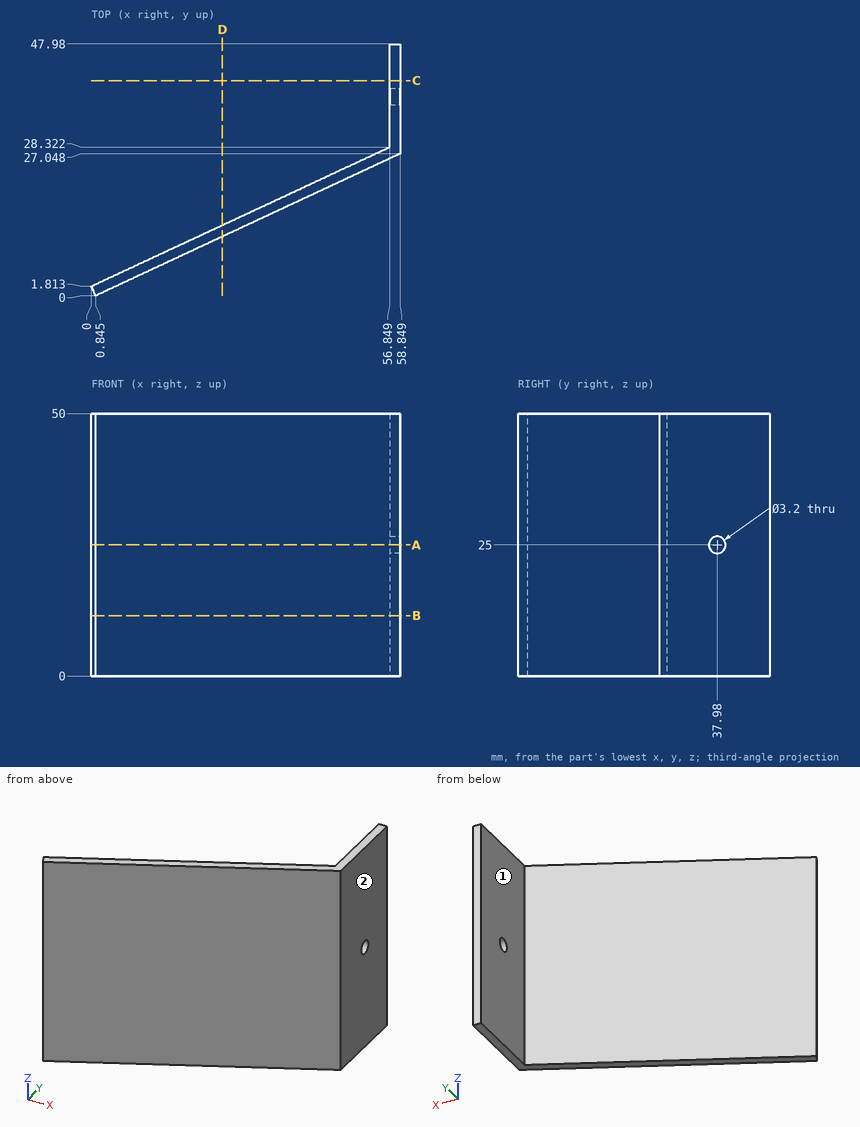
Input: dimensioned drawing with shaded views. Units: mm. Origin: part minimum x, y, z. A direction names the side the tool comes from. Coordinates: 2 decimals unless noted, no trailing zeros. Loops run counter-clockwise (first coordinate to the right, second up) from the corner with the lowest first, then second, coordinate; pieces in that order, holes last. Notation, with made-up numbers: M -3.5,50.25 L 14.5,50.25 A20 cw 14.5,66.25 Z; hole C 80,-16.5 d6. An arc over 180 degrees is marked long. One line per item, written item: value. Start each with the question number.
1) Cut plane D-D (x = 25). Return loops of the section in (y, z), then the cut area to 3 significant figures.
2) Cut plane B-B (z = 11.5). Return loops of the section in (x, y) (1 decimal), then the cut area to 3 significant figures.
3) Cut plane C-C (y = 41). Return loops of the section in (x, z).
4) Material intervals for L1, parallel to Y at x = 57.9, z = 25 (1 decimal); L2, parallel to Y at x = 57.65, z = 25; L3, parallel to X at y = 44.5, z = 13, sorted ascending. Write a range as from..to.
5) Pin query (flat end, axial travel): P1, Ø3, axis at x = 38, z = 15, coming from the -Y side; P2, Ø10, axis at x = 11, z = 30.5, coming from the -Y side; P3, Ø1.5, axis at y = 5.5, z = 20.5, coming from the +X side. Return the tip coordinate at first contact, or that it passes through.
6) Cut plane A-A (z = 25). Return loops of the section in (x, y) (1 decimal).
7) Reachability of the marked faces 1 and 2 from +Z, -Z, +X, -X, +Y, -Y: full face, straight path, thin tool, end or side. Return the list, or none.
Evaluation:
1. outline: M 11.26,0 L 13.47,0 L 13.47,50 L 11.26,50 Z
1. area: 110 mm^2
2. outline: M 0,1.8 L 0.8,0 L 58.8,27 L 58.8,48 L 56.8,48 L 56.8,28.3 Z
2. area: 167 mm^2
3. outline: M 56.85,0 L 58.85,0 L 58.85,50 L 56.85,50 Z
4. L1: 26.6..36.4, 39.6..48
4. L2: 26.49..36.38, 39.58..47.98
4. L3: 56.85..58.85
5. P1: y = 16.63
5. P2: y = 2.4
5. P3: x = 14.25
6. outline: M 0,1.8 L 0.8,0 L 58.8,27 L 58.8,36.4 L 56.8,36.4 L 56.8,28.3 Z; M 56.8,39.6 L 58.8,39.6 L 58.8,48 L 56.8,48 Z
7. face 1: +Z, -Z, -X, +Y
7. face 2: +Z, -Z, +X, +Y, -Y
